```python
from build123d import *

# Parameters (mm, degrees)
CYLINDER_R          = 3.765
CYLINDER_DEPTH      = 5
CYLINDER001_R       = 4.5
CYLINDER001_DEPTH   = 5
CUT_PLACEMENT_ANGLE = 90


with BuildPart() as cylinder:
    # Cylinder → Cylinder (new body)
    with BuildSketch(Plane.XY.offset(10)):
        Circle(CYLINDER_R)
    extrude(amount=CYLINDER_DEPTH)


with BuildPart() as obj1:
    # Cylinder001 → Cylinder001 (new body)
    with BuildSketch(Plane.XY.offset(10)):
        Circle(CYLINDER001_R)
    extrude(amount=CYLINDER001_DEPTH)

    # Cut: cut Cylinder
    add(cylinder.part, mode=Mode.SUBTRACT)


with BuildPart() as obj1_1:
    # Cut placement: moved
    add(obj1.part.moved(Location((-13, 0, 0))).rotate(Axis((-13, 0, 0), (0, 1, 0)), CUT_PLACEMENT_ANGLE))


solid = obj1_1.part
```
Design review of the part built by this model. Coordinates are the model's own, in mm. Round coordinates to 2 decimals unless told otherwise and drop trailing zeros. Write each loop counter-clockwise with the first axis right and the second up, starting at its lowest first coordinate (ties: lowest second). Pieces come first, ordered by that corner, then holes. Notation, with made-up numbers: (8.25, -3) -> (20.25, -3) arc R13 cw to (20.25, 18) -> close; hole circle Ø6 at (1.25, 38.25). An arc over 180 degrees is marked (long way). Write item = value, one per line. Start each with the question number.
1) Take a section at A-A, the plane z = 0. State the section outline as (x, y) points (3 decimals), plus the area to 3 significant figures.
2) Take a section at C-C, the plane x = -2.1. State the section outline as (y, z) points (3 decimals).
3) Clearance check with flat-ended pins moving along their axes: pin 1 (2 mm diameter, centred on y = -0.5, z = 2.5, fed in from +X) (3 decimals); pin 2 (1.5 mm diameter, centred on x = 0, z = -1.5, fed in from +Y); pin 3 (2 mm diameter, centred on x = -0.5, y = 1.5, fed in from +Z). State where each tip first meets the part, or that it passes through.
4) Mouldability with a two-part tool opening along Z and no side actions: class faces 1 (the face through (-0.535, 3.175, -2.024)), 2 (the face through (2, -4, 1)), 3 (the face through (-0.54, 4.46, 0.59)) as +Z half, -Z half, draft (parallel to the pull), parting line (faces both ways), or undercut.
5) Wall thickness on probe 1 along Y at (x, z) = (-1.7, 0) (3 decimals); probe 2 along Y at (x, z) = (1.5, -2.25); probe 3 along Z at (x, y) = (-2.55, 2.75): over which ranges is each line inside the solid? List them lowest first. Write a range as from..to.
Results list:
q1.outline = (-3, -4.5) -> (2, -4.5) -> (2, -3.765) -> (-3, -3.765) -> close; (-3, 3.765) -> (2, 3.765) -> (2, 4.5) -> (-3, 4.5) -> close
q1.area = 7.35 mm²
q2.outline = circle Ø9 at (0, 0); hole circle Ø7.53 at (0, 0)
q3.pin_1 = through
q3.pin_2 = 4.44
q3.pin_3 = 4.47
q4.face_1 = undercut
q4.face_2 = draft
q4.face_3 = parting line
q5.probe_1 = -4.5..-3.765, 3.765..4.5
q5.probe_2 = -3.9..-3.02, 3.02..3.9
q5.probe_3 = -3.56..-2.57, 2.57..3.56
